Model file for the job. Use its own axes, mm. A direction names the side the tool comes from. Round coordinates to 2 decimals unless told otherwise and drop trailing zeros. Loops run counter-clockwise (first coordinate to the right, second up) from the corner with the lowest first, then second, coordinate; pieces in that order, holes last. Notation, with made-up numbers: M 57,33 L 114,33 A32 cw 114,65 Z; hole C 26,74 d5. An arc over 180 degrees is marked long. Use a Markdown table: item, result. Add a question column.
Item 1: Saw through at B-B on z = -16. Write the cut outline in (x, y).
Item 2: Pin check, flat tips, straight feed: P1, Ø4, axis at x = -42, y = 7.5, coming from the +Z side; P2, Ø1.5, axis at x = 23.5, y = 4.5, coming from the -Z side; P3, Ø5, axis at x = -16, z = 0, coming from the +Y side; P4, Ø5, axis at y = 3, z = 26.5, coming from the -X side. Stop position of each tip, or through.
Item 3: Saw through at D-D on y = 5. Write the cut outline in (x, z), then the cut area to 3 significant figures.
Item 4: Wall check: L1, parallel to Z at x = -2.5, y = 4.25; L2, parallel to X at y = 5.5, z = -16; L3, parallel to Z at x = 1, y = 1.5. Give the ranges that are in metal, low to high. Write a range as from..to.
Item 5: Saw through at A-A on x = 0. Write the cut outline in (y, z).
Item 6: Tool access for faces 5 (the cylindrical face through (-36, 5, 23)), 6 (the cylindrical face through (0, 7, -55)): list every direction of +Z, -Z, +X, -X, +Y, -Y with a clear straight run to the whole face (end or side of a thin tool).
Item 7: Two-plate mould, pull along X, no slides. Class faces 1 (the cylindrical face through (-53.785, 4.93, -31.835)), 2 (the cylindrical face through (37.566, 4.93, 19.92)), 3 (the flat face through (52.006, 7.292, 30.298)), 4 (the cylindrical face through (48.58, 5.6, 25.84)): +X half, -X half, draft (parallel to the pull), parting line (faces both ways), or undercut.
Item 8: Saw through at C-C on x = 38.5. Write the cut outline in (y, z).
```python
from build123d import *

# Parameters (mm, degrees)
SKETCH1_R           = 62.5
SKETCH1_R_2         = 4
BOSS_EXTRUDE1_DEPTH = 10
SKETCH2_W           = 43.972180284
SKETCH2_H           = 8.711954994
CUT_EXTRUDE1_DEPTH  = 10
SKETCH3_R           = 2
CUT_EXTRUDE2_DEPTH  = 12
SKETCH4_R           = 2
CUT_EXTRUDE3_DEPTH  = 12
SKETCH5_R           = 2
CUT_EXTRUDE4_DEPTH  = 12
SKETCH6_R           = 11
CUT_EXTRUDE5_DEPTH  = 12
SKETCH7_R           = 1.5
CUT_EXTRUDE6_DEPTH  = 10


with BuildPart() as part:
    # Sketch1 → Boss-Extrude1 (new body)
    with BuildSketch(Plane(origin=(0, 0, 0), x_dir=(1, 0, 0), z_dir=(0, 1, 0))):
        with Locations(Location((0, 0, 0), (0, 0, 270))):
            Circle(SKETCH1_R)
        with Locations(Location((0, 46.188021535, 0), (0, 0, 270))):
            Circle(SKETCH1_R_2, mode=Mode.SUBTRACT)
        with Locations(Location((40, -23.094010768, 0), (0, 0, 270))):
            Circle(SKETCH1_R_2, mode=Mode.SUBTRACT)
        with Locations(Location((-40, -23.094010768, 0), (0, 0, 270))):
            Circle(SKETCH1_R_2, mode=Mode.SUBTRACT)
    extrude(amount=BOSS_EXTRUDE1_DEPTH)

    # Sketch2 → Cut-Extrude1 (cut)
    with BuildSketch(Plane(origin=(0, 10, 0), x_dir=(1, 0, 0), z_dir=(0, 1, 0))):
        Polygon((-39.581845605, -51.818275424), (-64.713070734, -8.289716646), (-77.687460418, -15.780484023), (-52.55623529, -59.309042801), align=None)
        Polygon((40.609652539, -50.038061596), (63.321086643, -10.700703814), (75.641288558, -17.813775707), (52.929854454, -57.151133488), align=None)
        with Locations((0.471086747, 64.543999032)):
            Rectangle(SKETCH2_W, SKETCH2_H)
    extrude(amount=-CUT_EXTRUDE1_DEPTH, mode=Mode.SUBTRACT)

    # Sketch3 → Cut-Extrude2 (cut)
    with BuildSketch(Plane(origin=(52.124355653, 0, 30.094010768), x_dir=(0.49999999999999983, 0, -0.8660254037844387), z_dir=(0.8660254037844387, 0, 0.49999999999999983))):
        with Locations((0.001973272, 5)):
            Circle(SKETCH3_R)
    extrude(amount=-CUT_EXTRUDE2_DEPTH, mode=Mode.SUBTRACT)

    # Sketch4 → Cut-Extrude3 (cut)
    with BuildSketch(Plane(origin=(-52.124355653, 0, 30.094010768), x_dir=(0.5000000000000002, 0, 0.8660254037844386), z_dir=(-0.8660254037844385, 0, 0.5000000000000001))):
        with Locations((-0.001973272, 5)):
            Circle(SKETCH4_R)
    extrude(amount=-CUT_EXTRUDE3_DEPTH, mode=Mode.SUBTRACT)

    # Sketch5 → Cut-Extrude4 (cut)
    with BuildSketch(Plane(origin=(0, 0, -60.188021535), x_dir=(-1, 0, 0), z_dir=(0, 0, -1))):
        with Locations((-0.001973272, 5)):
            Circle(SKETCH5_R)
    extrude(amount=-CUT_EXTRUDE4_DEPTH, mode=Mode.SUBTRACT)

    # Sketch6 → Cut-Extrude5 (cut)
    with BuildSketch(Plane(origin=(0, 10, 0), x_dir=(1, 0, 0), z_dir=(0, 1, 0))):
        with Locations(Location((0, 0, 0), (0, 0, 270))):
            Circle(SKETCH6_R)
    extrude(amount=-CUT_EXTRUDE5_DEPTH, mode=Mode.SUBTRACT)

    # Sketch7 → Cut-Extrude6 (cut)
    with BuildSketch(Plane(origin=(0, 10, 0), x_dir=(1, 0, 0), z_dir=(0, 1, 0))):
        with Locations(Location((-16, 0, 0), (0, 0, 270))):
            Circle(SKETCH7_R)
        with Locations(Location((0, 16, 0), (0, 0, 270))):
            Circle(SKETCH7_R)
        with Locations(Location((16, 0, 0), (0, 0, 270))):
            Circle(SKETCH7_R)
        with Locations(Location((0, -16, 0), (0, 0, 270))):
            Circle(SKETCH7_R)
    extrude(amount=-CUT_EXTRUDE6_DEPTH, mode=Mode.SUBTRACT)


solid = part.part
```
Entries:
| question | item | result |
|---|---|---|
| 1 | outline | M -60.42,0 L -1.5,0 L -1.5,10 L -60.42,10 Z; M 1.5,0 L 60.42,0 L 60.42,10 L 1.5,10 Z |
| 2 | P1 | z = 48.02 |
| 2 | P2 | z = -58.21 |
| 2 | P3 | y = 10 |
| 2 | P4 | x = -55.64 |
| 3 | outline | M -60.55,15.51 A62.5 ccw -16.84,-60.19 L -2,-60.19 L -2,-49.65 A4 cw long 2,-49.65 L 2,-60.19 L 16.84,-60.19 A62.5 ccw 60.55,15.51 L 53.13,28.36 L 44,23.09 A4 cw long 42,26.56 L 51.13,31.82 L 43.7,44.68 A62.5 ccw -43.7,44.68 L -51.13,31.82 L -42,26.56 A4 cw long -44,23.09 L -53.13,28.36 Z; hole C -16,0 d3; hole C 0,0 d22; hole C 0,-16 d3; hole C 0,16 d3; hole C 16,0 d3 |
| 3 | area | 11,400 mm2 |
| 4 | L1 | -60.19..-49.31, -43.07..-10.71, 10.71..62.45 |
| 4 | L2 | -60.42..-1.5, 1.5..60.42 |
| 4 | L3 | -60.19..-50.06, -42.32..-17.12, -14.88..-10.95, 10.95..14.88, 17.12..62.49 |
| 5 | outline | M 0,-60.19 L 3,-60.19 L 3,-50.19 L 0,-50.19 Z; M 0,-42.19 L 10,-42.19 L 10,-17.5 L 0,-17.5 Z; M 0,-14.5 L 10,-14.5 L 10,-11 L 0,-11 Z; M 0,11 L 10,11 L 10,14.5 L 0,14.5 Z; M 0,17.5 L 10,17.5 L 10,62.5 L 0,62.5 Z; M 7,-60.19 L 10,-60.19 L 10,-50.19 L 7,-50.19 Z |
| 6 | face 5 | +Y, -Y |
| 6 | face 6 | -Z |
| 7 | face 1 | -X half |
| 7 | face 2 | undercut |
| 7 | face 3 | +X half |
| 7 | face 4 | undercut |
| 8 | outline | M 0,-49.23 L 10,-49.23 L 10,19.39 L 0,19.39 Z; M 0,26.8 L 10,26.8 L 10,49.23 L 0,49.23 Z |
